Can you work these out from the model? Positions are in its coordinate system, mm. Face numbers are marked on the shaded views. Coordinates: 2 decimals unless noted, no trailing zeros. Order: outer loops, then holes, each group sorted by start corner. A loop starts at its lowest first (then second) coordinate and runs counter-clockwise, first axis right, second up. Notation, with made-up numbers: (-27.5, 5) -> (-6.5, 5) arc R17 cw to (-6.5, 36) -> close; hole circle Ø7 at (3, 9). An arc over 180 degrees is marked (long way). Write item = value, one per line.
```python
from build123d import *

# Parameters (mm, degrees)
SKETCH1_R           = 6.35
BOSS_EXTRUDE1_DEPTH = 25.4
SKETCH2_R           = 3.048
CUT_EXTRUDE1_DEPTH  = 8.636
SKETCH3_R           = 3.2385
CUT_EXTRUDE2_DEPTH  = 12.7


with BuildPart() as part:
    # Sketch1 → Boss-Extrude1 (new body)
    with BuildSketch(Plane(origin=(0, 0, 0), x_dir=(1, 0, 0), z_dir=(0, 1, 0))):
        Circle(SKETCH1_R)
    extrude(amount=BOSS_EXTRUDE1_DEPTH)

    # Sketch2 → Cut-Extrude1 (cut)
    with BuildSketch(Plane.XZ):
        Circle(SKETCH2_R)
    extrude(amount=-CUT_EXTRUDE1_DEPTH, mode=Mode.SUBTRACT)

    # Sketch3 → Cut-Extrude2 (cut)
    with BuildSketch(Plane(origin=(0, 25.4, 0), x_dir=(1, 0, 0), z_dir=(0, 1, 0))):
        Circle(SKETCH3_R)
    extrude(amount=-CUT_EXTRUDE2_DEPTH, mode=Mode.SUBTRACT)


solid = part.part
```
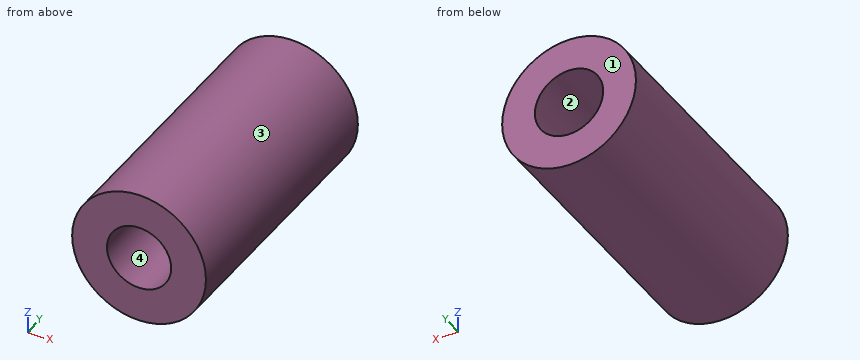
Item 1: I want a section at C-C, the plane y = 3. Please give me the cut outline in (x, z), plus the area to 3 significant figures.
A:
outline = circle Ø12.7 at (0, 0); hole circle Ø6.1 at (0, 0)
area = 97.5 mm2
Item 2: If I drill on probe 1 along X at (y, z) = (17.75, 0); probe 2 along Z at (x, y) = (0, 4.5), over which ranges is the centre line in solid material (lowest first)?
A:
probe_1 = -6.35 to -3.24, 3.24 to 6.35
probe_2 = -6.35 to -3.05, 3.05 to 6.35
Item 3: I'm going to push flat-ended pins straight in: P1, Ø5, axis at y = 8, z = 3, coming from the +X side; P2, Ø2, axis at y = 11, z = -2.5, coming from the -X side; P3, Ø5.5, axis at x = 0, z = 0, coming from the -Y side. Where does each tip first touch, or does it pass through?
A:
P1 = 6.33
P2 = -6.17
P3 = 8.64
Item 4: I want a section at A-A, the plane z = 0. Please give me the cut outline in (x, y), plus the area to 3 significant figures.
A:
outline = (-6.35, 0) -> (-3.05, 0) -> (-3.05, 8.64) -> (3.05, 8.64) -> (3.05, 0) -> (6.35, 0) -> (6.35, 25.4) -> (3.24, 25.4) -> (3.24, 12.7) -> (-3.24, 12.7) -> (-3.24, 25.4) -> (-6.35, 25.4) -> close
area = 188 mm2
Item 5: If we mould it in two halves opening along Z, with no side actions, what happens to the marked faces 1, 2, 3 and 4? For each: pulls with the +Z half, pulls with the -Z half, needs draft (parallel to the pull), parting line crosses it, or undercut.
A:
face_1 = needs draft
face_2 = undercut
face_3 = parting line crosses it
face_4 = undercut
Item 6: I want a section at D-D, the plane y = 9. Please give me the cut outline in (x, z), plus the area to 3 significant figures.
A:
outline = circle Ø12.7 at (0, 0)
area = 127 mm2
Item 7: I want a section at B-B, the plane x = 0. Please give me the cut outline in (y, z).
A:
outline = (0, -6.35) -> (25.4, -6.35) -> (25.4, -3.24) -> (12.7, -3.24) -> (12.7, 3.24) -> (25.4, 3.24) -> (25.4, 6.35) -> (0, 6.35) -> (0, 3.05) -> (8.64, 3.05) -> (8.64, -3.05) -> (0, -3.05) -> close
